from build123d import *

# Parameters (mm, degrees)
SKETCH1_R           = 7.825
SKETCH1_R_2         = 6.325
BOSS_EXTRUDE1_DEPTH = 12.75
BOSS_EXTRUDE2_START = -5.75
SKETCH1_2_R         = 7.825
BOSS_EXTRUDE2_DEPTH = 5.75
CUT_EXTRUDE1_DEPTH  = 5.75


with BuildPart() as part:
    # Sketch1 → Boss-Extrude1 (new body)
    with BuildSketch(Plane(origin=(0, 0, 0), x_dir=(1, 0, 0), z_dir=(0, 1, 0))):
        with Locations(Location((0, 0, 0), (0, 0, 270))):
            Circle(SKETCH1_R)
        with Locations(Location((0, 0, 0), (0, 0, 270))):
            Circle(SKETCH1_R_2, mode=Mode.SUBTRACT)
    extrude(amount=BOSS_EXTRUDE1_DEPTH)

    # Sketch1_2 → Boss-Extrude2 (add)
    with BuildSketch(Plane(origin=(0, 0, 0), x_dir=(1, 0, 0), z_dir=(0, 1, 0)).offset(BOSS_EXTRUDE2_START)):
        with Locations(Location((0, 0, 0), (0, 0, 270))):
            Circle(SKETCH1_2_R)
    extrude(amount=BOSS_EXTRUDE2_DEPTH)

    # Sketch2 → Cut-Extrude1 (cut)
    with BuildSketch(Plane.XZ.offset(5.75)):
        with BuildLine():
            Line((-2, 1.525), (2, 1.525))
            ThreePointArc((2, 1.525), (3.525, 0), (2, -1.525))
            Line((2, -1.525), (-2, -1.525))
            ThreePointArc((-2, -1.525), (-3.525, 0), (-2, 1.525))
        make_face()
    extrude(amount=-CUT_EXTRUDE1_DEPTH, mode=Mode.SUBTRACT)


solid = part.part
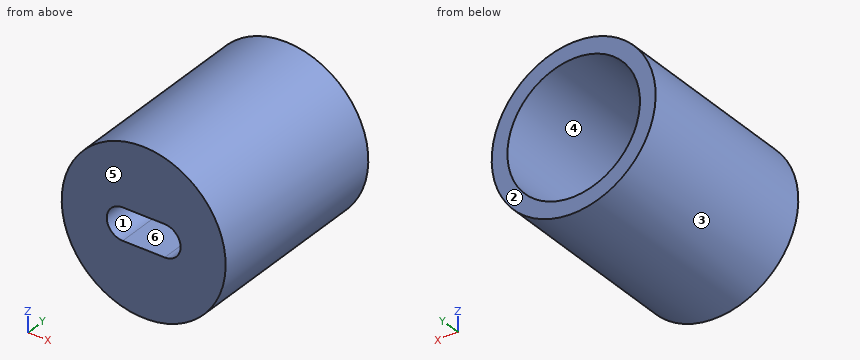
Work out the finished part from the listing and answer in its coordinate system (mm). Face numbers are marked on the shaded views. A direction names the side the tool comes from. Give positions to 0.01 mm unless a question says otherwise; leave off trailing zeros. Order: outer loops, then holes, each group sorted by start corner. A loop starts at its lowest first (then second) coordinate and runs counter-clockwise, first axis right, second up. Notation, with made-up numbers: (25, -23.5) -> (51, -23.5) arc R30 cw to (51, 6.5) -> close; hole circle Ø1 at (64, 16). An arc over 180 degrees is marked (long way). Answer as a JSON object with one key per item and string values. Group by question number.
1. Section B-B on z = 0 is taken. Determine the outline of the cut face in (x, y) (3 decimals).
2. Section C-C on y = -3.5 is taken. Determine the outline of the cut face in (x, z) (3 decimals), plus the area to 3 significant figures.
3. Section A-A on x = 0 is taken. Determine the outline of the cut face in (y, z) (3 decimals), plus the area to 3 significant figures.
4. A tool of negligible diameter and unlimited length cuts with its end or side. For the marked faces 1 and 2, from which of +Z, -Z, +X, -X, +Y, -Y can it reach the whole face along a straight path? Write none if from no direction.
5. Consider line 1 along X through (y, z) = (-4.25, 0) (3 decimals); line 2 along X through (y, z) = (10.25, 0) (3 decimals); line 3 along Z through (x, y) = (-1.5, 3.75). Determine where each line is inside the solid, lowest interval first. Write a range as [from, to].
6. Flat-ended cylindrical pins translate along their axes: pin 1 Ø1 at (x, y) = (1, -2.5) entering from -Z; pin 2 Ø2 at (x, y) = (-1.5, -1) entering from +Z. Find the tip coordinate at first contact, or state that the pin passes through.
7. The mould has two halves that part along Z. Classify the marked faces 3, 4, 5 and 6: released by +Z, released by -Z, zero draft, split by the parting line, or undercut.
8. Section D-D on z = 5.25 is taken. Determine the outline of the cut face in (x, y), plus the area to 3 significant figures.
Result sheet:
{
 "1": {"outline": "(-7.825, -5.75) -> (-3.525, -5.75) -> (-3.525, 0) -> (-6.325, 0) -> (-6.325, 12.75) -> (-7.825, 12.75) -> close; (3.525, -5.75) -> (7.825, -5.75) -> (7.825, 12.75) -> (6.325, 12.75) -> (6.325, 0) -> (3.525, 0) -> close"},
 "2": {"outline": "circle Ø15.65 at (0, 0); hole (-2, -1.525) -> (2, -1.525) arc R1.525 ccw to (2, 1.525) -> (-2, 1.525) arc R1.525 ccw to start", "area": "173 mm^2"},
 "3": {"outline": "(-5.75, -7.825) -> (12.75, -7.825) -> (12.75, -6.325) -> (0, -6.325) -> (0, -1.525) -> (-5.75, -1.525) -> close; (-5.75, 1.525) -> (0, 1.525) -> (0, 6.325) -> (12.75, 6.325) -> (12.75, 7.825) -> (-5.75, 7.825) -> close", "area": "111 mm^2"},
 "4": {"face 1": "+Y, -Y", "face 2": "+Z, -Z, +X, -X, +Y"},
 "5": {"line 1": "x = [-7.825, -3.525], [3.525, 7.825]", "line 2": "x = [-7.825, -6.325], [6.325, 7.825]", "line 3": "z = [-7.68, -6.14], [6.14, 7.68]"},
 "6": {"pin 1": "stops at z = -7.81", "pin 2": "stops at z = 7.81"},
 "7": {"face 3": "split by the parting line", "face 4": "undercut", "face 5": "zero draft", "face 6": "undercut"},
 "8": {"outline": "(-5.8, -5.75) -> (5.8, -5.75) -> (5.8, 12.75) -> (3.53, 12.75) -> (3.53, 0) -> (-3.53, 0) -> (-3.53, 12.75) -> (-5.8, 12.75) -> close", "area": "125 mm^2"}
}
